```python
from build123d import *

# Parameters (mm, degrees)
F1_DEPTH = 38.1


with BuildPart() as f1:
    # F0 (on Top) → F1 (new body)
    with BuildSketch(Plane.XY):
        with BuildLine():
            Line((-38.1, 25.4), (-38.1, 0))
            ThreePointArc((-38.1, 0), (0, -38.1), (38.1, 0))
            Line((38.1, 0), (38.1, 25.4))
            ThreePointArc((38.1, 25.4), (34.380256, 34.380256), (25.4, 38.1))
            Line((25.4, 38.1), (0, 38.1))
            Line((0, 38.1), (-25.4, 38.1))
            ThreePointArc((-25.4, 38.1), (-34.380256, 34.380256), (-38.1, 25.4))
        make_face()
        with BuildLine():
            ThreePointArc((22.849819, 8.417652), (0, -24.350998), (-22.849819, 8.417652))
            ThreePointArc((-22.849819, 8.417652), (-18.196877, 14.444923), (-10.932743, 16.727516))
            Line((-10.932743, 16.727516), (0, 16.727516))
            Line((0, 16.727516), (10.932743, 16.727516))
            ThreePointArc((10.932743, 16.727516), (18.196877, 14.444923), (22.849819, 8.417652))
        make_face(mode=Mode.SUBTRACT)
    extrude(amount=F1_DEPTH)


solid = f1.part
```
Here's how the part is built. I have some questions about the finished solid (model axes, mm). A direction names the side the tool comes from. Round coordinates to 2 decimals unless told otherwise and drop trailing zeros. Order: outer loops, then holes, each group sorted by start corner. A loop starts at its lowest first (then second) coordinate and runs counter-clockwise, first axis right, second up. Notation, with made-up numbers: (13, 33) -> (31, 33) arc R29 ccw to (31, 59) -> close; hole circle Ø5 at (-7.5, -25.75). An arc over 180 degrees is marked (long way). Use a Markdown table: item, result. Add a question column.
(1) For pin 1 Ø8 at (x, z) = (-22.5, 22) entering from -Y; pin 2 Ø8 at (y, z) = (-12, 33) entering from -X; pin 3 Ø1.5 at (x, z) = (25, 15.5) entering from -Y; pin 4 Ø6 at (x, z) = (-27, 18.5) entering from +Y, each with a flat end and sliding along its axis, tell me the tip position at first contact or that it passes through.
(2) Suppose I cut it at D-D, the plane x = -31. Please give me the cut outline in (y, z), and give its area (3 significant figures).
(3) If we mould it in two halves opening along Y, with no side actions, what happens to faces 1 (the face through (38.1, 13, 19)), 2 (the face through (18.108, 14.506, 18.783)), 3 (the face through (-0.84, -38.09, 18.78))? For each: released by +Y, released by -Y, zero draft, split by the parting line, or undercut.
(4) Suppose I cut it at A-A, the plane z = 13.5. Please give me the cut outline in (x, y).
(5) Suppose I cut it at C-C, the plane y = -8. Please give me the cut outline in (x, z).
(6) For faces 4 (the face through (0, 38.1, 19)), 5 (the face through (-18.29, 14.38, 18.78)), which set-ups out of +Z, -Z, +X, -X, +Y, -Y let a thin tool reach every point of the face, with its end or its side?
(7) Suppose I cut it at B-B, the plane x = 0. Please give me the cut outline in (y, z).
(8) I need wall thicknesses on line 1 along Y through (x, z) = (0, 9); line 2 along X through (y, z) = (-9, 19.5); line 3 along X through (y, z) = (-13, 34). Which ranges of each line are inside material? Lowest first, please.
Verdict:
| question | item | result |
|---|---|---|
| 1 | pin 1 | y = -33.31 |
| 1 | pin 2 | x = -37.25 |
| 1 | pin 3 | y = -29.39 |
| 1 | pin 4 | y = 38.1 |
| 2 | outline | (-22.15, 0) -> (36.8, 0) -> (36.8, 38.1) -> (-22.15, 38.1) -> close |
| 2 | area | 2,250 mm2 |
| 3 | face 1 | zero draft |
| 3 | face 2 | undercut |
| 3 | face 3 | released by -Y |
| 4 | outline | (-38.1, 0) arc R38.1 ccw to (38.1, 0) -> (38.1, 25.4) arc R12.7 ccw to (25.4, 38.1) -> (-25.4, 38.1) arc R12.7 ccw to (-38.1, 25.4) -> close; hole (-22.85, 8.42) arc R24.35 ccw (long way) to (22.85, 8.42) arc R12.7 ccw to (10.93, 16.73) -> (-10.93, 16.73) arc R12.7 ccw to start |
| 5 | outline | (-37.25, 0) -> (-23, 0) -> (-23, 38.1) -> (-37.25, 38.1) -> close; (23, 0) -> (37.25, 0) -> (37.25, 38.1) -> (23, 38.1) -> close |
| 6 | face 4 | +Z, -Z, +X, -X, +Y |
| 6 | face 5 | +Z, -Z |
| 7 | outline | (-38.1, 0) -> (-24.35, 0) -> (-24.35, 38.1) -> (-38.1, 38.1) -> close; (16.73, 0) -> (38.1, 0) -> (38.1, 38.1) -> (16.73, 38.1) -> close |
| 8 | line 1 | -38.1 to -24.35, 16.73 to 38.1 |
| 8 | line 2 | -37.02 to -22.63, 22.63 to 37.02 |
| 8 | line 3 | -35.81 to -20.59, 20.59 to 35.81 |
